```python
from build123d import *

# Parameters (mm, degrees)
BOSS_EXTRUDE1_DEPTH                            = 16
CBORE_FOR_6_SOCKET_HEAD_CAP_SCREW1_D           = 3.6576
CBORE_FOR_6_SOCKET_HEAD_CAP_SCREW1_DEPTH       = 9.398
CBORE_FOR_6_SOCKET_HEAD_CAP_SCREW1_CBORE_D     = 7.14502
CBORE_FOR_6_SOCKET_HEAD_CAP_SCREW1_CBORE_DEPTH = 2.54
CBORE_FOR_6_SOCKET_HEAD_CAP_SCREW1_TIP         = 1.0988539
FILLET1_R                                      = 0.75


with BuildPart() as part:
    # Sketch1 → Boss-Extrude1 (new, symmetric)
    with BuildSketch(Plane(origin=(0, 0, 0), x_dir=(0, 0, -1), z_dir=(1, 0, 0))):
        Polygon((0, 6.35), (3.175, 9.525), (6.35, 9.525), (6.35, -9.525), (0, -9.525), align=None)
    extrude(amount=BOSS_EXTRUDE1_DEPTH, both=True)

    # CBORE for #6 Socket Head Cap Screw1
    with Locations(Plane(origin=(0, 0, -6.35), x_dir=(-1, 0, 0), z_dir=(0, 0, -1))):
        with Locations((11.525, -5.025), (-11.525, 5.025), (-11.525, -5.025), (11.525, 5.025)):
            CounterBoreHole(CBORE_FOR_6_SOCKET_HEAD_CAP_SCREW1_D / 2, CBORE_FOR_6_SOCKET_HEAD_CAP_SCREW1_CBORE_D / 2, CBORE_FOR_6_SOCKET_HEAD_CAP_SCREW1_CBORE_DEPTH, depth=CBORE_FOR_6_SOCKET_HEAD_CAP_SCREW1_DEPTH)
            with Locations((0, 0, -(CBORE_FOR_6_SOCKET_HEAD_CAP_SCREW1_DEPTH + CBORE_FOR_6_SOCKET_HEAD_CAP_SCREW1_TIP / 2))):  # 118° drill point
                Cone(0, CBORE_FOR_6_SOCKET_HEAD_CAP_SCREW1_D / 2, CBORE_FOR_6_SOCKET_HEAD_CAP_SCREW1_TIP, mode=Mode.SUBTRACT)

    # Fillet1
    fillet1_edges = [part.edges().sort_by_distance(p)[0] for p in [
        (0, 6.35, 0),
        (0, -9.525, 0),
    ]]
    fillet(fillet1_edges, radius=FILLET1_R)


solid = part.part
```
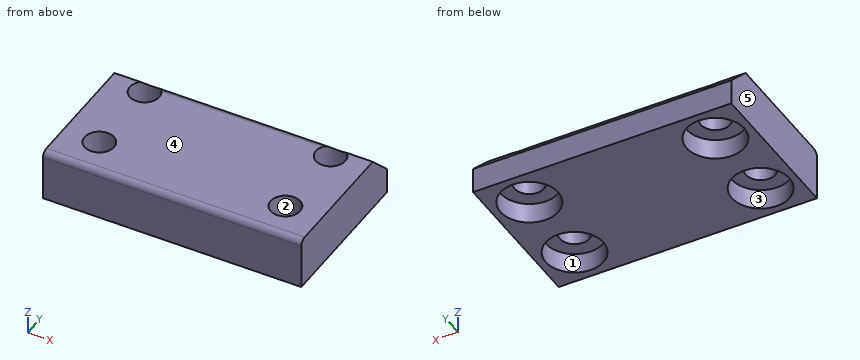
Part model, mm, in its own coordinate system. Face numbers are marked on the shaded views. A direction names the side the tool comes from. Round coordinates to 2 decimals unless told otherwise and drop trailing zeros. Write each loop counter-clockwise with the first axis right and the second up, starting at its lowest first coordinate (ties: lowest second). Pieces come first, ordered by that corner, then holes.
Item 1: Cut at C-C, the plane x = -12. Give the cut face in (y, z) (3 decimals).
Results:
outline: (-9.525, -6.35) - (-8.566, -6.35) - (-8.566, -3.81) - (-6.791, -3.81) - (-6.791, 0) - (-8.775, 0) arc R0.75 ccw to (-9.525, -0.75) - close; (-3.259, -3.81) - (-1.484, -3.81) - (-1.484, -6.35) - (1.484, -6.35) - (1.484, -3.81) - (3.259, -3.81) - (3.259, 0) - (-3.259, 0) - close; (6.791, -3.81) - (8.566, -3.81) - (8.566, -6.35) - (9.525, -6.35) - (9.525, -3.175) - (6.791, -0.441) - close
Item 2: Cut at A-A, the plane y = 4.5. Give the cut face in (x, z), plus the area to 3 significant figures.
Results:
outline: (-16, -6.35) - (-15.06, -6.35) - (-15.06, -3.81) - (-13.28, -3.81) - (-13.28, 0) - (-16, 0) - close; (-9.77, -3.81) - (-7.99, -3.81) - (-7.99, -6.35) - (7.99, -6.35) - (7.99, -3.81) - (9.77, -3.81) - (9.77, 0) - (-9.77, 0) - close; (13.28, -3.81) - (15.06, -3.81) - (15.06, -6.35) - (16, -6.35) - (16, 0) - (13.28, 0) - close
area: 141 mm2
Item 3: Two-plate mould, pull along X, no slides. Class the marked faces 3, 4 and 5: +X half, -X half, draft (parallel to the pull), parting line (faces both ways), or undercut.
Results:
face 3: undercut
face 4: draft
face 5: -X half
Item 4: Drop flat-ended pins along their axis: pin 1 Ø6 at (x, y) = (-11.525, -5.025) entering from -Z; pin 2 Ø3 at (x, y) = (11.525, 5.025) entering from -Z; pin 3 Ø1 at (x, z) = (-3, -1) entering from +Y. Give the stop position or say it passes through.
Results:
pin 1: stops at z = -3.81
pin 2: passes through
pin 3: stops at y = 7.85
Item 5: Which spindle directions (+Z, -Z, +X, -X, +Y, -Y) get a long thin tool onto all of the face, cutting with end or side? Do the marked faces 1 and 2. Say none if no direction does.
Results:
face 1: -Z
face 2: +Z, -Z
Item 6: Probe L1, parallel to X at y = 5.25, z = -5; L2, parallel to Y at x = 13, z = -1.5 (3 decimals); L3, parallel to X at y = -4.25, z = -4. List the from-to ranges inside material, lowest first.
Results:
L1: x = -16 to -15.09, -7.96 to 7.96, 15.09 to 16
L2: y = -9.525 to -6.106, -3.944 to 3.944, 6.106 to 7.85
L3: x = -16 to -15.01, -8.04 to 8.04, 15.01 to 16
Item 7: Cut at B-B, the plane z = -2.25. Give the cut face in (x, y) (3 decimals).
Results:
outline: (-16, -9.525) - (16, -9.525) - (16, 8.6) - (-16, 8.6) - close; hole circle Ø3.658 at (-11.525, -5.025); hole circle Ø3.658 at (-11.525, 5.025); hole circle Ø3.658 at (11.525, -5.025); hole circle Ø3.658 at (11.525, 5.025)
Item 8: Cut at D-D, the plane y = 2.5. Give the cut face in (x, z), plus the area to 3 significant figures.
Results:
outline: (-16, -6.35) - (-14.05, -6.35) - (-14.05, -3.81) - (-9, -3.81) - (-9, -6.35) - (9, -6.35) - (9, -3.81) - (14.05, -3.81) - (14.05, -6.35) - (16, -6.35) - (16, 0) - (-16, 0) - close
area: 178 mm2
